```python
from build123d import *

# Parameters (mm, degrees)
F0_R     = 1.7526
F0_W     = 59.9948
F0_H     = 89.0524
F1_DEPTH = 10.9982
F3_DEPTH = 3.175
F4_R     = 2.54


with BuildPart() as f1:
    # F0 (on Top) → F1 (new body)
    with BuildSketch(Plane.XY):
        Polygon((29.9974, 54.5338), (-29.9974, 54.5338), (-29.9974, 74.549), (-40.005, 74.549), (-40.005, 54.5338), (-40.005, -54.5338), (-40.005, -74.549), (-29.9974, -74.549), (-29.9974, -54.5338), (29.9974, -54.5338), (29.9974, -74.549), (40.005, -74.549), (40.005, -54.5338), (40.005, 54.5338), (40.005, 74.549), (29.9974, 74.549), align=None)
        with Locations((-16.1798, -49.53)):
            Circle(F0_R, mode=Mode.SUBTRACT)
        with Locations((16.1798, -49.53)):
            Circle(F0_R, mode=Mode.SUBTRACT)
        with Locations((-16.1798, 49.53)):
            Circle(F0_R, mode=Mode.SUBTRACT)
        Rectangle(F0_W, F0_H, mode=Mode.SUBTRACT)
        with Locations((16.1798, 49.53)):
            Circle(F0_R, mode=Mode.SUBTRACT)
    extrude(amount=F1_DEPTH)

    # F2 (on face) → F3 (join)
    with BuildSketch(Plane.XY.offset(10.9982)):
        with BuildLine():
            ThreePointArc((-29.9974, 67.275193), (-35.106164, 64.756103), (-40.005, 61.849782))
            Line((-40.005, 61.849782), (-40.005, -61.849782))
            ThreePointArc((-40.005, -61.849782), (-35.106164, -64.756103), (-29.9974, -67.275193))
            Line((-29.9974, -67.275193), (-29.9974, -54.5338))
            Line((-29.9974, -54.5338), (-29.9974, -44.5262))
            Line((-29.9974, -44.5262), (-29.9974, 44.5262))
            Line((-29.9974, 44.5262), (-29.9974, 54.5338))
            Line((-29.9974, 54.5338), (-29.9974, 67.275193))
        make_face()
        with BuildLine():
            Line((29.9974, 67.275193), (29.9974, 54.5338))
            Line((29.9974, 54.5338), (29.9974, 44.5262))
            Line((29.9974, 44.5262), (29.9974, -44.5262))
            Line((29.9974, -44.5262), (29.9974, -54.5338))
            Line((29.9974, -54.5338), (29.9974, -67.275193))
            ThreePointArc((29.9974, -67.275193), (35.106164, -64.756103), (40.005, -61.849782))
            Line((40.005, -61.849782), (40.005, 61.849782))
            ThreePointArc((40.005, 61.849782), (35.106164, 64.756103), (29.9974, 67.275193))
        make_face()
    extrude(amount=F3_DEPTH)

    # F4
    f4_edges = [f1.edges().sort_by_distance(p)[0] for p in [
        (29.9974, 44.5262, 5.4991),
        (-29.9974, 44.5262, 5.4991),
        (29.9974, 54.5338, 5.4991),
        (-29.9974, 54.5338, 5.4991),
        (-29.9974, 74.549, 5.4991),
        (-40.005, 74.549, 5.4991),
        (29.9974, 74.549, 5.4991),
        (40.005, 74.549, 5.4991),
        (29.9974, -74.549, 5.4991),
        (40.005, -74.549, 5.4991),
        (-29.9974, -74.549, 5.4991),
        (-40.005, -74.549, 5.4991),
        (-29.9974, -54.5338, 5.4991),
        (29.9974, -54.5338, 5.4991),
        (29.9974, -44.5262, 5.4991),
        (-29.9974, -44.5262, 5.4991),
    ]]
    fillet(f4_edges, radius=F4_R)


solid = f1.part
```
Source: CAD feature listing. Evaluate the final solid. Frame: model axes, mm. A direction names the side the tool comes from. Give positions to 0.01 mm unless a question says otherwise; leave off trailing zeros. Loops run counter-clockwise (first coordinate to the right, second up) from the corner with the lowest first, then second, coordinate; pieces in that order, holes last. Notation, with made-up numbers: (50, 32) - (85, 32) arc R11 cw to (85, 44) - close; hole circle Ø5 at (80.5, -7.75). An arc over 180 degrees is marked (long way). Use CSV: the item, a comma, the result in double quotes.
1) Pin query (flat end, axial travel): P1, Ø3, axis at x = -16.18, y = -49.53, coming from the +Z side; P2, Ø8, axis at x = 25, z = 7.5, coming from the +Y side; P3, Ø6, axis at x = -15, z = 6.5, coming from the +Y side; P4, Ø4, axis at x = 16.18, y = 49.53, coming from the +Z side. Return the tip coordinate at first contact, or that it passes through.
Worked out:
P1,"passes through"
P2,"stops at y = 55.06"
P3,"stops at y = 54.53"
P4,"stops at z = 11"
2) Set-up query: faces 5 (the flat face through (-35, -70, 10.998)), 6 (the flat face through (0, -44.526, 5)), 7 (the cylindrical face through (35.04, -64.79, 12.56)). Return all of +Z, -Z, +X, -X, +Y, -Y with unobstructed straight access to the full face (end or side cutting, diameter ignored); none if empty.
Worked out:
face 5,"+Z, -X, -Y"
face 6,"+Z, -Z"
face 7,"+Z, +X, -Y"
3) Cut plane D-D (y = -65). Output: boundary loops of the cut face in (x, z) (1 decimal), and give its area (3 significant figures).
Worked out:
outline,"(-40, 0) - (-30, 0) - (-30, 14.2) - (-34.7, 14.2) - (-34.7, 11) - (-40, 11) - close; (30, 0) - (40, 0) - (40, 11) - (34.7, 11) - (34.7, 14.2) - (30, 14.2) - close"
area,"250 mm^2"
4) Cut plane B-B (y = 49.53). Output: boundary loops of the cut face in (x, z) (3 decimals), and give its area (3 significant figures).
Worked out:
outline,"(-40.005, 0) - (-17.932, 0) - (-17.932, 10.998) - (-29.997, 10.998) - (-29.997, 14.173) - (-40.005, 14.173) - close; (-14.427, 0) - (14.427, 0) - (14.427, 10.998) - (-14.427, 10.998) - close; (17.932, 0) - (40.005, 0) - (40.005, 14.173) - (29.997, 14.173) - (29.997, 10.998) - (17.932, 10.998) - close"
area,"866 mm^2"
5) Mould query, pull axis Y, two halves, no side actions, for faces 1 (the cylindrical face through (15.8, -51.24, 5.42)), 2 (the cylindrical face through (-35.04, 64.79, 12.56)), 3 (the flat face through (29.997, 1, 7)), 4 (the flat face through (0, -51, 10.998)). Classes: +Y half, -Y half, draft (parallel to the pull), parting line (faces both ways), or undercut.
Worked out:
face 1,"undercut"
face 2,"+Y half"
face 3,"undercut"
face 4,"draft"
6) Cut plane C-C (x = -26). Output: boundary loops of the cut face in (y, z).
Worked out:
outline,"(-54.53, 0) - (-44.53, 0) - (-44.53, 11) - (-54.53, 11) - close; (44.53, 0) - (54.53, 0) - (54.53, 11) - (44.53, 11) - close"
7) Cut plane A-A (z = 12.5). Output: boundary loops of the cut face in (x, y) (3 decimals).
Worked out:
outline,"(-40.005, -61.85) arc R73.66 ccw to (-29.997, -67.275) - (-29.997, 67.275) arc R73.66 ccw to (-40.005, 61.85) - close; (29.997, -67.275) arc R73.66 ccw to (40.005, -61.85) - (40.005, 61.85) arc R73.66 ccw to (29.997, 67.275) - close"
8) Line query: line 1 (X direction, y = 22.5, z = 7) (3 decimals); line 2 (Y direction, x = -10, z = 8); line 3 (Y direction, x = 15, z = 4.5). Output: solid intervals per line, ascending.
Worked out:
line 1,"x = -40.005 to -29.997, 29.997 to 40.005"
line 2,"y = -54.53 to -44.53, 44.53 to 54.53"
line 3,"y = -54.53 to -50.83, -48.23 to -44.53, 44.53 to 48.23, 50.83 to 54.53"
